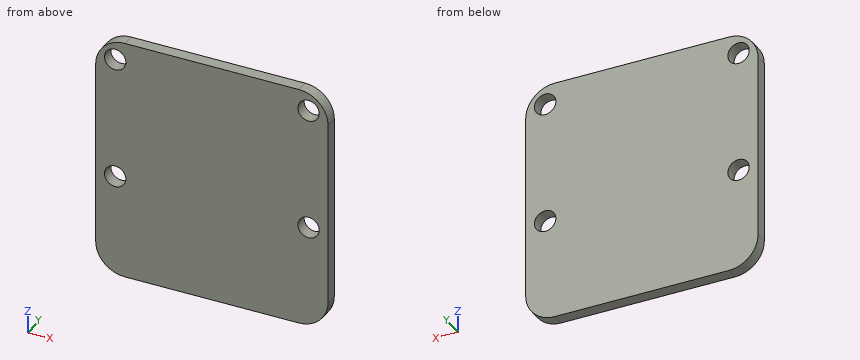
Autodesk Inventor part; units mm, degrees
ref_plane "YZ Plane" through (0, 0, 0) normal (1, 0, 0) x (0, 1, 0)
ref_plane "XZ Plane" through (0, 0, 0) normal (0, 1, 0) x (-1, 0, 0)
ref_plane "XY Plane" through (0, 0, 0) normal (0, 0, 1) x (1, 0, 0)
sketch "Sketch1" plane through (0, 0, 0) normal (0, 1, 0) x (-1, 0, 0)
  line L0 (11.931, 12.5) -> (-11.931, 12.5)
  line L1 (-11.931, 12.5) -> (-11.931, -12.5)
  line L2 (-11.931, -12.5) -> (11.931, -12.5)
  line L3 (11.931, -12.5) -> (11.931, 12.5)
  line L4 (11.931, 12.5) -> (-11.931, -12.5) construction
  line L5 (-11.931, 12.5) -> (11.931, -12.5) construction
  point P0 (0, 0)
  point P1 (-29, 11.5)
  point P2 (-29, -11.5)
  dimension "d0" = 23.862
  dimension "d1" = 25
extrude "Extrusion1" add sketch "Sketch1" against normal blind 1.27
fillet "Fillet1" radius 3 4 edges at (-11.931, -0.635, 12.5) (11.931, -0.635, 12.5) (11.931, -0.635, -12.5) (-11.931, -0.635, -12.5)
sketch "Sketch3" plane through (0, 0, 0) normal (0, 1, 0) x (1, 0, 0)
  line L0 (9.931, -10.5) -> (-9.931, -10.5) construction
  line L1 (-9.931, -10.5) -> (-9.931, 2) construction
  line L2 (-9.931, 2) -> (9.931, 2) construction
  line L3 (9.931, 2) -> (9.931, -10.5) construction
  line L4 (-8.931, -12.5) -> (8.931, -12.5)
  line L5 (11.931, -9.5) -> (11.931, 9.5)
  line L6 (-11.931, 9.5) -> (-11.931, -9.5)
  point P0 (0, 0)
  dimension "d16" = 2
  dimension "d17" = 2
  dimension "d18" = 2
  dimension "d19" = 14.5
hole "Hole2" at (9.931, 0, 10.5) at (9.931, 0, -2) at (-9.931, 0, -2) at (-9.931, 0, 10.5) direction (0, -1, 0) diameter 2.2 end through all
equation "\"d0\" = PiCameraLength"
equation "\"d1\" = PiCameraWidth"
equation "\"d4\" = PiZeroWHeight"
equation "\"PiZeroWHeight\" = 1.27"
equation "\"PiCameraWidth\" = 25"
equation "\"PiCameraLength\" = 23.862"
properties part number "PiCameraWithMechanicalLayout" material "LCP Plastic"
Model file for the job. Use its own axes, mm. Give positions to 0.01 mm unless a question says otherwise; leave off trailing zeros. Order: outer loops, then holes, each group sorted by start corner. A loop starts at its lowest first (then second) coordinate and runs counter-clockwise, first axis right, second up.
1) Wall check: probe 1 along X at (y, z) = (-0.25, -2); probe 2 along Z at (x, y) = (-9.75, -0.55) (3 decimals); probe 3 along X at (y, z) = (-0.1, 11.5). Give the ranges that are in metal, low to high.
2) Saw through at C-C, the plane z = 10.5. Write the cut outline in (x, y), then the cut area to 3 significant figures.
3) Saw through at B-B, the plane y = -1. Write the cut outline in (x, z), then the cut area to 3 significant figures.
4) Saw through at A-A, the plane z = -2. Write the cut outline in (x, y), then the cut area to 3 significant figures.
5) Pin check, flat tip, straight feed: pin 1 (1.3 mm diameter, centred on x = 9.931, z = -2, fed in from -Y). Stop position of the tip, or through.
Computed:
1. probe 1: x = -11.93 to -11.03, -8.83 to 8.83, 11.03 to 11.93
1. probe 2: z = -12.386 to -3.085, -0.915 to 9.415, 11.585 to 12.386
1. probe 3: x = -11.17 to -10.39, -9.47 to 9.47, 10.39 to 11.17
2. outline: (-11.76, -1.27) - (-11.03, -1.27) - (-11.03, 0) - (-11.76, 0) - close; (-8.83, -1.27) - (8.83, -1.27) - (8.83, 0) - (-8.83, 0) - close; (11.03, -1.27) - (11.76, -1.27) - (11.76, 0) - (11.03, 0) - close
2. area: 24.3 mm2
3. outline: (-11.93, -9.5) arc R3 ccw to (-8.93, -12.5) - (8.93, -12.5) arc R3 ccw to (11.93, -9.5) - (11.93, 9.5) arc R3 ccw to (8.93, 12.5) - (-8.93, 12.5) arc R3 ccw to (-11.93, 9.5) - close; hole circle Ø2.2 at (-9.93, -2); hole circle Ø2.2 at (-9.93, 10.5); hole circle Ø2.2 at (9.93, -2); hole circle Ø2.2 at (9.93, 10.5)
3. area: 574 mm2
4. outline: (-11.93, -1.27) - (-11.03, -1.27) - (-11.03, 0) - (-11.93, 0) - close; (-8.83, -1.27) - (8.83, -1.27) - (8.83, 0) - (-8.83, 0) - close; (11.03, -1.27) - (11.93, -1.27) - (11.93, 0) - (11.03, 0) - close
4. area: 24.7 mm2
5. pin 1: passes through
